Source: CAD feature listing. Evaluate the final solid. Frame: model axes, mm. A direction names the side the tool comes from. Round coordinates to 2 decimals unless told otherwise and drop trailing zeros. Write each loop counter-clockwise with the first axis right and the second up, starting at its lowest first coordinate (ties: lowest second). Pieces come first, ordered by that corner, then holes. Notation, with made-up numbers: M 28,8.5 L 68,8.5 A17 ccw 68,39.5 Z; hole C 32,23.25 d4. An arc over 180 degrees is marked long. Use a Markdown table: item, result.
```python
from build123d import *

# Parameters (mm, degrees)
F1_DEPTH = 25.4


with BuildPart() as f1:
    # F0 (on Top) → F1 (new body)
    with BuildSketch(Plane.XY):
        with BuildLine():
            ThreePointArc((593.7185342312, 713.2225054204), (54.903166967, 490.0378726846), (-168.2814657688, -48.7774945796))
            Line((-168.2814657688, -48.7774945796), (593.7185342312, -48.7774945796))
            Line((593.7185342312, -48.7774945796), (1355.7185342312, -48.7774945796))
            ThreePointArc((1355.7185342312, -48.7774945796), (1132.5339014953, 490.0378726846), (593.7185342312, 713.2225054204))
        make_face()
        with BuildLine():
            Line((578.9150146893, 27.4225054204), (558.8869975048, 27.4225054204))
            Line((558.8869975048, 27.4225054204), (-87.8349853107, 27.4225054204))
            ThreePointArc((-87.8349853108, 27.4225054204), (-14.5690429068, 267.9366722959), (140.4555796865, 465.8819404232))
            Line((140.4555796865, 465.8819404232), (578.9150146893, 27.4225054204))
        make_face(mode=Mode.SUBTRACT)
        with BuildLine():
            ThreePointArc((1049.2347336709, 463.8887048602), (1202.6992993376, 266.6017497128), (1275.2720537731, 27.4225054204))
            Line((1275.2720537731, 27.4225054204), (612.7685342312, 27.4225054204))
            Line((612.7685342312, 27.4225054204), (1049.2347336709, 463.8887048602))
        make_face(mode=Mode.SUBTRACT)
        with BuildLine():
            Line((578.9150146893, 636.8627141372), (578.9150146893, 81.3040334204))
            Line((578.9150146893, 81.3040334204), (386.5735172011, 273.5404429351))
            Line((386.5735172011, 273.5404429351), (169.7362173216, 490.2592712796))
            ThreePointArc((169.7362173216, 490.2592712796), (362.4040406687, 596.8348078651), (578.9150146893, 636.8627141372))
        make_face(mode=Mode.SUBTRACT)
        with BuildLine():
            Line((1019.9483620731, 488.4838699888), (917.7654260406, 386.3009339562))
            Line((917.7654260406, 386.3009339562), (612.7685342312, 81.3040421469))
            Line((612.7685342312, 81.3040421469), (612.7685342312, 636.757871029))
            ThreePointArc((612.7685342312, 636.757871029), (828.3774912664, 595.6267371595), (1019.9483620731, 488.4838699888))
        make_face(mode=Mode.SUBTRACT)
    extrude(amount=F1_DEPTH)


solid = f1.part
```
Q1. Line query: L1, parallel to X at y = 529.5, z = 24.25; L2, parallel to Y at x = 371.5, z = 11.25; L3, parallel to X at y = 335, z = 19.75. Output: solid intervals per line, ascending.
Results are:
| item | result |
|---|---|
| L1 | 97.49 to 225.05, 578.92 to 612.77, 962.39 to 1089.94 |
| L2 | -48.78 to 27.42, 234.84 to 288.61, 600.02 to 680.1 |
| L3 | -64.58 to 25.36, 271.34 to 325.08, 578.92 to 612.77, 866.46 to 920.35, 1162.08 to 1252.02 |
Q2. Mould query, pull axis X, two halves, no side actions, for faces 1 (the cylindrical face through (1201.073, 269.722, 12.522)), 2 (the flat face through (583, 253, 25.4)), 3 (the cylindrical face through (610.47, 713.04, 12.52)). Classes: +X half, -X half, draft (parallel to the pull), parting line (faces both ways), or undercut.
Results are:
| item | result |
|---|---|
| face 1 | undercut |
| face 2 | draft |
| face 3 | parting line |
Q3. Section A-A on y = 45. Return loops of the section in (x, z).
Results are:
| item | result |
|---|---|
| outline | M -162.49,0 L -85.64,0 L -85.64,25.4 L -162.49,25.4 Z; M 561.34,0 L 630.35,0 L 630.35,25.4 L 561.34,25.4 Z; M 1273.08,0 L 1349.93,0 L 1349.93,25.4 L 1273.08,25.4 Z |
Q4. Section D-D on y = 407. Return loops of the section in (x, z), plus the area to 3 significant figures.
Results are:
| item | result |
|---|---|
| outline | M -16.95,0 L 81.28,0 L 81.28,25.4 L -16.95,25.4 Z; M 199.34,0 L 253.04,0 L 253.04,25.4 L 199.34,25.4 Z; M 578.92,0 L 612.77,0 L 612.77,25.4 L 578.92,25.4 Z; M 938.46,0 L 992.35,0 L 992.35,25.4 L 938.46,25.4 Z; M 1106.15,0 L 1204.38,0 L 1204.38,25.4 L 1106.15,25.4 Z |
| area | 8,580 mm^2 |
Q5. Section B-B on x = 648. Return loops of the section in (y, z).
Results are:
| item | result |
|---|---|
| outline | M -48.78,0 L 27.42,0 L 27.42,25.4 L -48.78,25.4 Z; M 62.65,0 L 116.54,0 L 116.54,25.4 L 62.65,25.4 Z; M 634.87,0 L 711.29,0 L 711.29,25.4 L 634.87,25.4 Z |
Q6. Reachability of faces 4 (the flat face through (356.62, 249.72, 12.52)), 5 (the flat face through (583, 253, 0)) from +Z, -Z, +X, -X, +Y, -Y: full face, straight path, thin tool, end or side. Return the list, or none.
Results are:
| item | result |
|---|---|
| face 4 | +Z, -Z |
| face 5 | -Z, +X, -X, +Y, -Y |
Q7. First-contact query: pin 1 Ø2 at (y, z) = (198, 9.5) entering from +X; pin 2 Ø10 at (y, z) = (576.5, 21.5) entering from -X; pin 3 Ø2 at (y, z) = (256.5, 20) entering from +X. Flat tips, straight axial feed; report the tip coordinate or a pass-through.
Results are:
| item | result |
|---|---|
| pin 1 | x = 1314.99 |
| pin 2 | x = 151.11 |
| pin 3 | x = 1292.33 |
Q8. Section C-C on z = 20.25. Return loops of the section in (x, y).
Results are:
| item | result |
|---|---|
| outline | M -168.28,-48.78 L 1355.72,-48.78 A762 ccw Z; hole M -87.83,27.42 L 578.92,27.42 L 140.46,465.88 A685.8 ccw Z; hole M 169.74,490.26 L 578.92,81.3 L 578.92,636.86 A685.8 ccw Z; hole M 612.77,27.42 L 1275.27,27.42 A685.8 ccw 1049.23,463.89 Z; hole M 612.77,81.3 L 1019.95,488.48 A685.8 ccw 612.77,636.76 Z |
